Could you check a few things on this drawing? It's one solid part, dimensions in mm from its lowest x, y, z. Coordinates: 2 decimals unless noted, no trailing zeros. Write each loop counter-clockwise with the first axis right and the second up, starting at its lowest first coordinate (ties: lowest second). Pieces come first, ordered by that corner, then holes. Notation, with made-up numbers: (6, -36.75) - (27, -36.75) arc R12 cw to (27, -29.75) - close; hole circle Ø8 at (-9, -27.5). An arc over 180 degrees is marked (long way). Answer as a JSON object with one key per item and string values. Group by question number.
1) If we section it at A-A (y = 25): Write out the boundary of the cut face in (x, z).
2) If we section it at C-C (z = 4.1): Write out the boundary of the cut face in (x, y).
3) Will this pin go through, and if not, where does the flat tip stop? pin 1 Ø25 at (x, y) = (25, 25) entering from -Z.
4) Please list where these lines run through material, in increasing order: line 1 along Y through (x, z) = (25, 1.95); line 2 along Y through (x, z) = (31, 0.45); line 3 along X through (y, z) = (20, 1.4).
5) We'd pull the mould along X, two halves only. Please class the marked faces 1 and 2: released by +X, released by -X, zero draft, split by the parting line, or undercut.
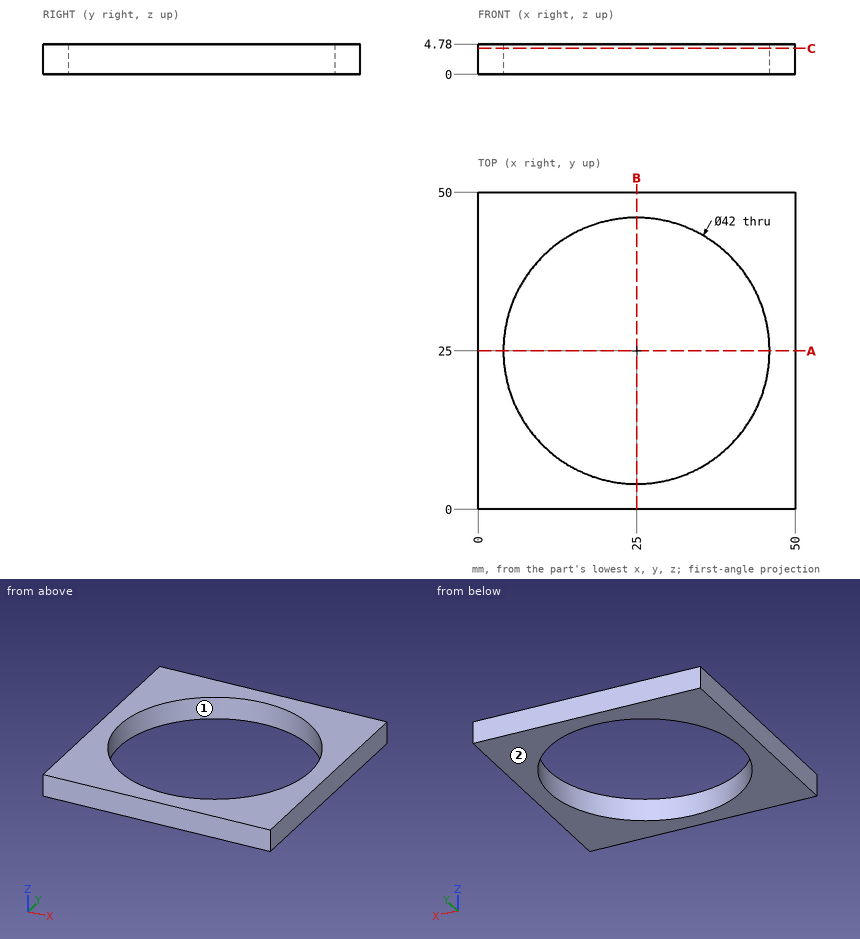
Here are the results:
{
 "1": {"outline": "(0, 0) - (4, 0) - (4, 4.78) - (0, 4.78) - close; (46, 0) - (50, 0) - (50, 4.78) - (46, 4.78) - close"},
 "2": {"outline": "(0, 0) - (50, 0) - (50, 50) - (0, 50) - close; hole circle Ø42 at (25, 25)"},
 "3": {"pin 1": "passes through"},
 "4": {"line 1": "y = 0 to 4, 46 to 50", "line 2": "y = 0 to 4.88, 45.12 to 50", "line 3": "x = 0 to 4.6, 45.4 to 50"},
 "5": {"face 1": "undercut", "face 2": "zero draft"}
}
